from build123d import *

# Parameters (mm, degrees)
SKETCH1_R           = 8.74
BOSS_EXTRUDE2_DEPTH = 6.35
FILLET1_R           = 10
SKETCH2_R           = 4.5
CUT_EXTRUDE1_DEPTH  = 71.132527363
SKETCH3_R           = 1.25
CUT_EXTRUDE2_DEPTH  = 71.132527363
CUT_EXTRUDE5_DEPTH  = 71.132527363
FILLET2_R           = 2
FILLET3_R           = 2


with BuildPart() as part:
    # Sketch1 → Boss-Extrude2 (new body)
    with BuildSketch(Plane(origin=(0, 0, 0), x_dir=(1, 0, 0), z_dir=(0, 1, 0))):
        with BuildLine():
            ThreePointArc((-7.16851449, -5), (-8.74, 0), (-7.16851449, 5))
            Line((-7.16851449, 5), (-32.16851449, 5))
            ThreePointArc((-32.16851449, 5), (-46.487760751, 16.45991775), (-54.187285312, 33.10587371))
            add(Edge.make_bspline(
                [(-54.187285312, 33.10587371), (-69.799584501, 0), (-54.187285312, -33.10587371)],
                knots=[1.078170572, 1.078170572, 1.078170572, 2.063422082, 2.063422082, 2.063422082], degree=2, weights=[1, 0.88109407, 1]))
            ThreePointArc((-54.187285312, -33.10587371), (-46.487760751, -16.45991775), (-32.16851449, -5))
            Line((-32.16851449, -5), (-7.16851449, -5))
        make_face()
        Circle(SKETCH1_R)
        with BuildLine():
            Line((32.16851449, 5), (7.16851449, 5))
            ThreePointArc((7.16851449, 5), (8.337877927, 2.620570868), (8.74, 0))
            ThreePointArc((8.74, 0), (8.337877927, -2.620570868), (7.16851449, -5))
            Line((7.16851449, -5), (32.16851449, -5))
            ThreePointArc((32.16851449, -5), (46.487760751, -16.45991775), (54.187285312, -33.10587371))
            add(Edge.make_bspline(
                [(54.187285312, -33.10587371), (69.799584501, 0), (54.187285312, 33.10587371)],
                knots=[4.219763225, 4.219763225, 4.219763225, 5.205014735, 5.205014735, 5.205014735], degree=2, weights=[1, 0.88109407, 1]))
            ThreePointArc((54.187285312, 33.10587371), (46.487760751, 16.45991775), (32.16851449, 5))
        make_face()
    extrude(amount=BOSS_EXTRUDE2_DEPTH)

    # Fillet1
    fillet1_edges = [part.edges().sort_by_distance(p)[0] for p in [
        (-32.16851449, 3.175, -5),
        (-7.16851449, 3.175, -5),
        (7.16851449, 3.175, -5),
        (32.16851449, 3.175, -5),
        (32.16851449, 3.175, 5),
        (7.16851449, 3.175, 5),
        (-7.16851449, 3.175, 5),
        (-32.16851449, 3.175, 5),
    ]]
    fillet(fillet1_edges, radius=FILLET1_R)

    # Sketch2 → Cut-Extrude1 (cut, through all)
    with BuildSketch(Plane(origin=(0, 6.35, 0), x_dir=(1, 0, 0), z_dir=(0, 1, 0))):
        with Locations(Location((0, 0, 0), (0, 0, 270))):
            Circle(SKETCH2_R)
    extrude(amount=-CUT_EXTRUDE1_DEPTH, mode=Mode.SUBTRACT)

    # Sketch3 → Cut-Extrude2 (cut, through all)
    with BuildSketch(Plane(origin=(0, 6.35, 0), x_dir=(1, 0, 0), z_dir=(0, 1, 0))):
        with Locations(Location((-6.2464, 0, 0), (0, 0, 270))):
            Circle(SKETCH3_R)
        with Locations(Location((3.1232, 5.409541082, 0), (0, 0, 270))):
            Circle(SKETCH3_R)
        with Locations(Location((3.1232, -5.409541082, 0), (0, 0, 270))):
            Circle(SKETCH3_R)
    extrude(amount=-CUT_EXTRUDE2_DEPTH, mode=Mode.SUBTRACT)

    # Sketch4 → Cut-Extrude5 (cut, through all)
    with BuildSketch(Plane(origin=(0, 6.35, 0), x_dir=(1, 0, 0), z_dir=(0, 1, 0))):
        with BuildLine():
            add(Edge.make_bspline(
                [(-54.07815408, -18.814509315), (-54.878953653, -15.771750191), (-55.485617126, -12.659616872), (-56.296145207, -6.364958437), (-56.5, -3.182494687), (-56.5, 3.182494687), (-56.296145207, 6.364958437), (-55.485617126, 12.659616872), (-54.878953653, 15.771750191), (-54.07815408, 18.814509315)],
                knots=[0, 0, 0, 0, 0.25, 0.25, 0.5, 0.5, 0.75, 0.75, 1, 1, 1, 1], degree=3))
            ThreePointArc((-54.07815408, 18.814509315), (-46.738015221, 9.226749217), (-37.112695661, 1.935932696))
            Line((-37.112695661, 1.935932696), (-37.112695661, -1.935932696))
            ThreePointArc((-37.112695661, -1.935932696), (-46.738015221, -9.226749217), (-54.07815408, -18.814509315))
        make_face()
        with BuildLine():
            ThreePointArc((37.112695661, -1.935932696), (46.738015221, -9.226749217), (54.07815408, -18.814509315))
            add(Edge.make_bspline(
                [(54.07815408, -18.814509315), (54.878953653, -15.771750191), (55.485617126, -12.659616872), (56.296145207, -6.364958437), (56.5, -3.182494687), (56.5, 3.182494687), (56.296145207, 6.364958437), (55.485617126, 12.659616872), (54.878953653, 15.771750191), (54.07815408, 18.814509315)],
                knots=[0, 0, 0, 0, 0.25, 0.25, 0.5, 0.5, 0.75, 0.75, 1, 1, 1, 1], degree=3))
            ThreePointArc((54.07815408, 18.814509315), (46.738015221, 9.226749217), (37.112695661, 1.935932696))
            Line((37.112695661, 1.935932696), (37.112695661, -1.935932696))
        make_face()
    extrude(amount=-CUT_EXTRUDE5_DEPTH, mode=Mode.SUBTRACT)

    # Fillet2
    fillet2_edges = [part.edges().sort_by_distance(p)[0] for p in [
        (-37.112695661, 3.175, 1.935932696),
        (-37.112695661, 3.175, -1.935932696),
        (-54.07815408, 3.175, 18.814509315),
        (-54.07815408, 3.175, -18.814509315),
    ]]
    fillet(fillet2_edges, radius=FILLET2_R)

    # Fillet3
    fillet3_edges = [part.edges().sort_by_distance(p)[0] for p in [
        (54.07815408, 3.175, 18.814509315),
        (54.07815408, 3.175, -18.814509315),
        (37.112695661, 3.175, -1.935932696),
        (37.112695661, 3.175, 1.935932696),
    ]]
    fillet(fillet3_edges, radius=FILLET3_R)


solid = part.part
Work out the finished part from the listing and answer in its coordinate system (mm). A direction names the side the tool comes from. Give positions to 0.01 mm unless a question says otherwise; leave off trailing zeros. Write each loop counter-clockwise with the first axis right and the second up, starting at its lowest first coordinate (ties: lowest second). Pieces come first, ordered by that corner, then holes. Notation, with made-up numbers: (-4, 84) - (22, 84) arc R29 ccw to (22, 118) - close; hole circle Ø3 at (63, 46.25). An arc over 180 degrees is marked (long way). One line per item, written item: value. Start each with the question number.
1. For a pull along Z with two mould halves and no side action, classify faces 1 (the cylindrical face through (-32.25, 3.22, -5.32)), 2 (the flat face through (20, 3, 5)), 3 (the cylindrical face through (45.37, 3.22, 7.92)) as +Z half, -Z half, draft (parallel to the pull), parting line (faces both ways), or undercut.
2. Find section D-D (x = 45). Write down the section's boundary in (y, z).
3. Find section B-B (z = 12). State how many separate pieces and enclosed holes the cut face has, then the cut area to 3 significant figures.
4. Find section A-A (x = 0). Write down the section's boundary in (y, z).
5. Consider probe 1 along X at (y, z) = (1.5, 0); probe 2 along X at (y, z) = (3, 10); probe 3 along X at (y, z) = (3.75, -3.5). Determine where each line is inside the solid, lowest interval first.
6. Given pin 1 (0.5 mm diameter, centred on y = 2.5, z = 0.5, fed in from +X); pin 2 (3 mm diameter, centred on x = 23.5, y = 3.5, fed in from +Z); pin 3 (3 mm diameter, centred on x = 23.5, y = 4.5, fed in from -Z), each flat-ended and moving along its own axis, determine where each tip first touches the part or whether it passes through.
7. For faces 4 (the cylindrical face through (8.117, 3.219, -5.498)), 5 (the flat face through (5, 0, 0)), 6 (the cylindrical face through (-32.32, 3.22, 5.34)), 7 (the cylindrical face through (-45.37, 3.22, 7.92)), 8 (the flat face through (5, 6.35, 0)), determine the directions among +Z, -Z, +X, -X, +Y, -Y from which every point of the face is accessible in a straight line to the end or side of a thin tool.
Geometry results:
1. face 1: -Z half
1. face 2: +Z half
1. face 3: undercut
2. outline: (0, -14.67) - (6.35, -14.67) - (6.35, -7.59) - (0, -7.59) - close; (0, 7.59) - (6.35, 7.59) - (6.35, 14.67) - (0, 14.67) - close
3. separate pieces: 4
3. enclosed holes: 0
3. area: 152 mm2
4. outline: (0, -8.74) - (6.35, -8.74) - (6.35, -4.5) - (0, -4.5) - close; (0, 4.5) - (6.35, 4.5) - (6.35, 8.74) - (0, 8.74) - close
5. probe 1: -61.5 to -56.5, -37.11 to -7.5, -5 to -4.5, 4.5 to 37.11, 56.5 to 61.5
5. probe 2: -60.87 to -55.83, -47.5 to -40.12, 40.12 to 47.5, 55.83 to 60.87
5. probe 3: -61.42 to -56.42, -39.68 to -2.83, 2.83 to 39.68, 56.42 to 61.42
6. pin 1: x = 61.5
6. pin 2: z = 5
6. pin 3: z = -5
7. face 4: -Z, +Y, -Y
7. face 5: +Z, -Z, +X, -X, -Y
7. face 6: +Z, +Y, -Y
7. face 7: +Y, -Y
7. face 8: +Z, -Z, +X, -X, +Y
